Autodesk Inventor part; units mm, degrees
ref_plane "YZ Plane" through (0, 0, 0) normal (1, 0, 0) x (0, 1, 0)
ref_plane "XZ Plane" through (0, 0, 0) normal (0, 1, 0) x (-1, 0, 0)
ref_plane "XY Plane" through (0, 0, 0) normal (0, 0, 1) x (1, 0, 0)
sketch "Sketch1" plane through (0, 0, 0) normal (1, 0, 0) x (0, 1, 0)
  line L0 (0, 0) -> (147, 0)
  line L1 (147, 0) -> (147, 110)
  line L2 (147, 110) -> (0, 110)
  line L3 (0, 110) -> (0, 0)
  circle A0 centre (124.75, 106.25) radius 1
  circle A1 centre (124.75, 3.75) radius 1
  circle A2 centre (22.25, 3.75) radius 1
  circle A3 centre (22.25, 106.25) radius 1
  circle A4 centre (84.4635, 28.1525) radius 1.5
  circle A5 centre (84.4635, 81.8475) radius 1.5
  circle A6 centre (62.5365, 81.8475) radius 1.5
  circle A7 centre (62.5365, 28.1525) radius 1.5
  dimension "d0" = 102.5
  dimension "d1" = 102.5
  dimension "d2" = 2
  dimension "d3" = 110
  dimension "d4" = 147
  dimension "d5" = 22.25
  dimension "d6" = 22.25
  dimension "d7" = 3.75
  dimension "d8" = 3.75
  dimension "d24" = 3
  dimension "d25" = 3
  dimension "d26" = 3
  dimension "d27" = 3
  dimension "d28" = 53.695
  dimension "d29" = 21.927
  dimension "d30" = 28.1525
  dimension "d31" = 28.1525
  dimension "d32" = 62.5365
  dimension "d33" = 62.5365
extrude "Extrusion1" add sketch "Sketch1" along normal blind 5
sketch "Sketch2" plane through (5, 0, 0) normal (1, 0, 0) x (0, 0, -1)
  circle A0 centre (-55, 73.5) radius 11.125
  line L0 (-110, 0) -> (0, 0)
  line L1 (-110, 147) -> (-110, 0)
  point P0 (-55, 0)
  point P1 (-110, 73.5)
  dimension "d11" = 22.25
extrude "Extrusion2" cut sketch "Sketch2" against normal up to surface (5 mm away)
ref_plane "Work Plane1" through (0, 73.5, 0) normal (0, -1, 0) x (1, 0, 0)
sketch "Sketch3" plane through (0, 73.5, 0) normal (0, -1, 0) x (1, 0, 0)
  line L0 (5, 66.125) -> (5, 43.875)
  line L1 (0, 55) -> (5, 55) construction
  line L2 (0, 43.875) -> (0, 66.125)
  circle A0 centre (4, 67.125) radius 2.5
  point P0 (0, 0)
  dimension "d17" = 5
  dimension "d22" = 1
  dimension "d23" = 1
revolve "Revolution1" cut sketch "Sketch3" angle 360 about axis through (0, 73.5, 55) along (1, 0, 0)
equation "\"d1\" = d0"
equation "\"d5\" = d6"
equation "\"d7\" = d8"
equation "\"d30\" = d31"
equation "\"d32\" = d33"
properties part number "front plate"
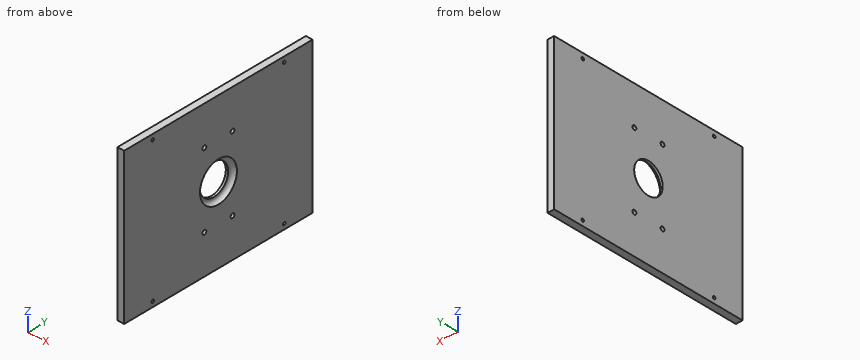
For this review, take the finished solid that the model builds, in its own axes (mm). Round coordinates to 2 decimals unless told otherwise and drop trailing zeros. Order: outer loops, then holes, each group sorted by start corner. A loop starts at its lowest first (then second) coordinate and runs counter-clockwise, first axis right, second up. Notation, with made-up numbers: M 63.25,52.5 L 85.25,52.5 A16 cw 85.25,76.5 Z; hole C 1,50.5 d5. An arc over 180 degrees is marked long. Use a Markdown table: item, result. Add a question column.
Item 1: To check wall thickness, follow line 1 along Z through (x, y) = (1.1, 22.25); line 2 along Z through (x, y) = (0.95, 73.5) (3 decimals); line 3 along Z through (x, y) = (2.4, 23). State the ranges of each line that lie inside material, in increasing order.
Item 2: Insertion check: pin 1 (1.2 mm diameter, centred on y = 22.25, z = 106.25, fed in from +X). The pin has a flat end and moves straight along its axis. Give the tip position at first contact, or say it passes through.
Item 3: Add section B-B, the plane x = 4. State how many separate pieces and enclosed holes the cut face has, then the cut area to 3 significant figures.
Item 4: Add section C-C, the plane y = 73.5. Give the boundary of the cut face in (x, z) (3 decimals).
Item 5: Add section A-A, the plane z = 55. Give the boundary of the cut face in (x, y) (3 decimals).
Geometry results:
| question | item | result |
|---|---|---|
| 1 | line 1 | z = 0 to 2.75, 4.75 to 105.25, 107.25 to 110 |
| 1 | line 2 | z = 0 to 43.875, 66.125 to 110 |
| 1 | line 3 | z = 0 to 3.09, 4.41 to 105.59, 106.91 to 110 |
| 2 | pin 1 | passes through |
| 3 | separate pieces | 1 |
| 3 | enclosed holes | 9 |
| 3 | area | 15,500 mm² |
| 4 | outline | M 0,0 L 5,0 L 5,40.584 A2.5 cw 1.709,43.875 L 0,43.875 Z; M 0,66.125 L 1.709,66.125 A2.5 cw 5,69.416 L 5,110 L 0,110 Z |
| 5 | outline | M 0,0 L 5,0 L 5,59.084 A2.5 cw 1.709,62.375 L 0,62.375 Z; M 0,84.625 L 1.709,84.625 A2.5 cw 5,87.916 L 5,147 L 0,147 Z |
